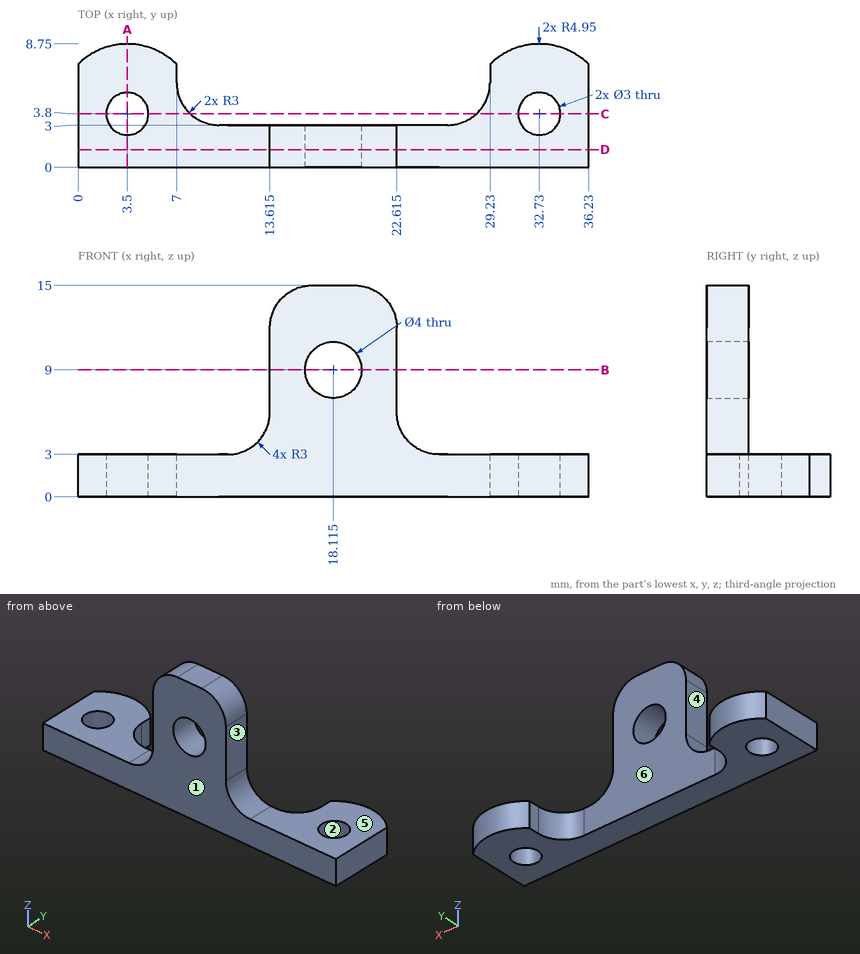
Design review of the part shown in the three views and the two pictorial views. Dimensions are in mm from the part's minimum x, y and z. A direction names the side the tool comes from. Round coordinates to 2 decimals unless told otherwise and drop trailing zeros. Loops run counter-clockwise (first coordinate to the right, second up) from the corner with the lowest first, then second, coordinate; pieces in that order, holes last. Notation, with made-up numbers: (86.5, 31.5) -> (92.5, 31.5) arc R18 ccw to (92.5, 58.5) -> close; hole circle Ø6 at (84, 47). An arc over 180 degrees is marked (long way). Answer as a JSON object with one key per item and string values. Group by question number.
1) We need section D-D on y = 1.25. Write out the cut boundary in (x, z) (1 decimal).
2) For line 1 (X direction, y = 4.25, z = 1.5); line 2 (X direction, y = 2.3, z = 9) (1 decimal); line 3 (Y direction, x = 22.5, z = 8.75), list the stretches that pass through material, from the lowest coordinate up. Write a range as [from, to].
3) We need section A-A on x = 3.5. Write out the cut boundary in (y, z).
4) Mouldability with a two-part tool opening along Y and no side actions: class the marked faces 1, 2 and 3 as released by +Y, released by -Y, zero draft, split by the parting line, or undercut.
5) We need section B-B on z = 9. Write out the cut boundary in (x, y) (1 decimal).
6) For the marked faces 4, 5 and 6, list the 3-axis set-ups (+Z, -Z, +X, -X, +Y, -Y) from which the entire face can be reached by the end or side of a thin tool; tool diameter is ignored.
7) For pin 1 Ø1.5 at (y, z) = (2, 12) entering from -X (3 decimals); pin 2 Ø5 at (y, z) = (5, 11.5) entering from +X (3 decimals); pin 3 Ø1 at (x, z) = (22, 9.5) entering from +Y, all flat-tipped, find the tip position at first contact; note any pin that passes through.
8) We need section C-C on y = 3.8. Write out the cut boundary in (x, z).
Result set:
{
 "1": {"outline": "(0, 0) -> (36.2, 0) -> (36.2, 3) -> (25.6, 3) arc R3 cw to (22.6, 6) -> (22.6, 12) arc R3 ccw to (19.6, 15) -> (16.6, 15) arc R3 ccw to (13.6, 12) -> (13.6, 6) arc R3 cw to (10.6, 3) -> (0, 3) -> close; hole circle Ø4 at (18.1, 9)"},
 "2": {"line 1": "[0, 2.07], [4.93, 7.56], [28.67, 31.3], [34.16, 36.23]", "line 2": "[13.6, 16.1], [20.1, 22.6]", "line 3": "[0, 3]"},
 "3": {"outline": "(0, 0) -> (2.3, 0) -> (2.3, 3) -> (0, 3) -> close; (5.3, 0) -> (8.75, 0) -> (8.75, 3) -> (5.3, 3) -> close"},
 "4": {"face 1": "released by -Y", "face 2": "undercut", "face 3": "zero draft"},
 "5": {"outline": "(13.6, 0) -> (16.1, 0) -> (16.1, 3) -> (13.6, 3) -> close; (20.1, 0) -> (22.6, 0) -> (22.6, 3) -> (20.1, 3) -> close"},
 "6": {"face 4": "+Z, -X, +Y, -Y", "face 5": "+Z, +X, +Y, -Y", "face 6": "+Z, -Z, +Y"},
 "7": {"pin 1": "x = 13.615", "pin 2": "x = 22.615", "pin 3": "y = 3"},
 "8": {"outline": "(0, 0) -> (2, 0) -> (2, 3) -> (0, 3) -> close; (5, 0) -> (7.96, 0) -> (7.96, 3) -> (5, 3) -> close; (28.27, 0) -> (31.23, 0) -> (31.23, 3) -> (28.27, 3) -> close; (34.23, 0) -> (36.23, 0) -> (36.23, 3) -> (34.23, 3) -> close"}
}
